from build123d import *

# Parameters (mm, degrees)
SKETCH1_W                   = 19.05
SKETCH1_H                   = 19.05
EXTRUDE1_DEPTH              = 19.05
F_29_0_136_DIAMETER_HOLE1_D = 3.4544
EXTRUDE2_DEPTH              = 1
EXTRUDE2_DEPTH_BACK         = 20.05
F_29_0_136_DIAMETER_HOLE3_D = 3.4544


with BuildPart() as part:
    # Sketch1 → Extrude1 (new body)
    with BuildSketch(Plane.XY):
        Rectangle(SKETCH1_W, SKETCH1_H)
    extrude(amount=EXTRUDE1_DEPTH)

    # #29 (0.136) Diameter Hole1 (through all)
    with Locations(Plane.ZY.offset(9.525)):
        with Locations((9.525, 0)):
            Hole(F_29_0_136_DIAMETER_HOLE1_D / 2)

    # Sketch7 → Extrude2 (cut, two sides)
    with BuildSketch(Plane.XY.offset(19.05)) as extrude2_sk:
        with BuildLine():
            Line((9.525, -9.525), (9.525, 0))
            ThreePointArc((9.525, 0), (9.353814185, -4.774759033), (8.841135768, -9.525))
            Line((8.841135768, -9.525), (9.525, -9.525))
        make_face()
        with BuildLine():
            ThreePointArc((8.841135768, 9.525), (9.353814185, 4.774759033), (9.525, 0))
            Line((9.525, 0), (9.525, 9.525))
            Line((9.525, 9.525), (8.841135768, 9.525))
        make_face()
    extrude(amount=EXTRUDE2_DEPTH, mode=Mode.SUBTRACT)
    extrude(extrude2_sk.sketch, amount=-EXTRUDE2_DEPTH_BACK, mode=Mode.SUBTRACT)

    # #29 (0.136) Diameter Hole3 (through all)
    with Locations(Plane(origin=(-4.445, 0, 19.05), x_dir=(1, 0, 0), z_dir=(0, 0, 1))):
        with Locations((0, 0)):
            Hole(F_29_0_136_DIAMETER_HOLE3_D / 2)


solid = part.part
Input: part model. Units: mm. Frame: model coordinates. Give positions to 0.01 mm unless a question says otherwise; leave off trailing zeros. Write each loop counter-clockwise with the first axis right and the second up, starting at its lowest first coordinate (ties: lowest second). Pieces come first, ordered by that corner, then holes. Notation, with made-up numbers: (-16, 63) -> (11, 63) arc R30 ccw to (11, 102) -> close; hole circle Ø4 at (37, 39). An arc over 180 degrees is marked (long way). Use one line per item in the form item = value. Start each with the question number.
1) Section query B-B on x = 4.25. Return the cut outline in (y, z) (3 decimals), then the cut area to 3 significant figures.
2) Pin query (flat end, axial travel): pin 1 (3 mm diameter, centred on x = -4.445, y = 0, fed in from +Z); pin 2 (5 mm diameter, centred on y = 7.5, z = 2.5, fed in from +X). Return the tip coordinate at first contact, or that it passes through.
3) Section query A-A on z = 10. Return the cut outline in (x, y) (3 decimals).
4) Section query D-D on y = 6.75. Return the cut outline in (x, z) (3 decimals), then the cut area to 3 significant figures.
5) Section query C-C on z = 4. Return the cut outline in (x, y) (3 decimals).
6) Ray query, probe 1 along X at (y, z) = (0, 2.75) (3 decimals); probe 2 along Y at (x, z) = (-4.5, 8.5) (3 decimals); probe 3 along X at (y, z) = (-1.5, 6.5) (3 decimals). Return the intervals inside material, ascending. Write a range as from..to.
7) Draft query along Y for faces 1 (the cylindrical face through (-6.04, -0.66, 4.7)), 2 (the flat face through (0, 0, 19.05)), 3 (the flat face through (0, -9.525, 9)), 4 (the cylindrical face through (2.638, -1.532, 8.728)). Return one class per face: pulls with the +Y half, pulls with the -Y half, needs draft (parallel to the pull), parting line crosses it, or undercut.
Outcome:
q1.outline = (-9.525, 0) -> (9.525, 0) -> (9.525, 19.05) -> (-9.525, 19.05) -> close; hole circle Ø3.454 at (0, 9.525)
q1.area = 354 mm^2
q2.pin_1 = through
q2.pin_2 = 9.34
q3.outline = (-9.525, -9.525) -> (8.841, -9.525) arc R66.675 ccw to (9.504, -1.661) -> (-3.97, -1.661) arc R1.727 cw to (-4.92, -1.661) -> (-9.525, -1.661) -> close; (-9.525, 1.661) -> (-4.92, 1.661) arc R1.727 cw to (-3.97, 1.661) -> (9.504, 1.661) arc R66.675 ccw to (8.841, 9.525) -> (-9.525, 9.525) -> close
q4.outline = (-9.525, 0) -> (9.182, 0) -> (9.182, 19.05) -> (-9.525, 19.05) -> close
q4.area = 356 mm^2
q5.outline = (-9.525, -9.525) -> (8.841, -9.525) arc R66.675 ccw to (8.841, 9.525) -> (-9.525, 9.525) -> close; hole circle Ø3.454 at (-4.445, 0)
q6.probe_1 = -9.525..-6.172, -2.718..9.525
q6.probe_2 = -9.525..-1.726, 1.726..9.525
q6.probe_3 = -9.525..-5.301, -3.589..9.508
q7.face_1 = undercut
q7.face_2 = needs draft
q7.face_3 = pulls with the -Y half
q7.face_4 = undercut
